Work out the finished part from the listing and answer in its coordinate system (mm). Face numbers are marked on the shaded views. A direction names the side the tool comes from. Coordinates: 2 decimals unless noted, no trailing zeros. Write each loop counter-clockwise with the first axis right and the second up, starting at its lowest first coordinate (ties: lowest second). Pieces come first, ordered by that corner, then holes. Notation, with made-up numbers: (2.5, -9.75) - (22.5, -9.75) arc R26 cw to (22.5, 8.25) - close; hole circle Ø8 at (-23, 84.25). An arc over 180 degrees is marked (long way). Use one line per item in the form item = value. Start each with the question number.
Item 1: A cutting plane is placed at B-B (z = 5). Write down the section's boundary in (x, y).
Item 2: For the marked faces 1 and 2, determine the directions among +Z, -Z, +X, -X, +Y, -Y from which every point of the face is accessible in a straight line to the end or side of a thin tool.
Item 3: Consider probe 1 along X at (y, z) = (-1.5, 5); probe 2 along Y at (x, z) = (-7.5, 7); probe 3 along Y at (x, z) = (1.5, 7.75). Determine where each line is inside the solid, lowest interval first.
Item 4: Given pin 1 (1 mm diameter, centred on x = 9.5, z = 6.5, fed in from -Y); pin 2 (1.8 mm diameter, centred on x = 2.5, z = 5, fed in from +Y) (3 decimals), each flat-ended and moving along its own axis, determine where each tip first touches the part or whether it passes through.
Item 5: A cutting plane is placed at A-A (y = 0). Write down the section's boundary in (x, z), then the cut area to 3 significant figures.
Item 6: A cutting plane is placed at C-C (x = -7.5). Write down the section's boundary in (y, z).
Item 7: A cutting plane is placed at D-D (y = -3.25). Write down the section's boundary in (x, z), then the cut area to 3 significant figures.
from build123d import *

# Parameters (mm, degrees)
SKETCH1_W           = 30
SKETCH1_H           = 10
BOSS_EXTRUDE1_DEPTH = 10
SKETCH2_R           = 1
CUT_EXTRUDE1_DEPTH  = 19.708286934
SKETCH4_R           = 1
CUT_EXTRUDE3_DEPTH  = 21.615528128
SKETCH3_R           = 1
BOSS_EXTRUDE2_DEPTH = 5


with BuildPart() as part:
    # Sketch1 → Boss-Extrude1 (new body)
    with BuildSketch(Plane.XY):
        Rectangle(SKETCH1_W, SKETCH1_H)
    extrude(amount=BOSS_EXTRUDE1_DEPTH)

    # Sketch2 → Cut-Extrude1 (cut, through all)
    with BuildSketch(Plane.XY.offset(10)):
        with Locations((-7.5, 0)):
            Circle(SKETCH2_R)
        with Locations((7.5, 0)):
            Circle(SKETCH2_R)
    extrude(amount=-CUT_EXTRUDE1_DEPTH, mode=Mode.SUBTRACT)

    # Sketch4 → Cut-Extrude3 (cut, through all)
    with BuildSketch(Plane(origin=(0, 5, 0), x_dir=(1, 0, 0), z_dir=(0, 1, 0))):
        with Locations(Location((-2.5, -5, 0), (0, 0, 270))):
            Circle(SKETCH4_R)
        with Locations(Location((2.5, -5, 0), (0, 0, 270))):
            Circle(SKETCH4_R)
    extrude(amount=-CUT_EXTRUDE3_DEPTH, mode=Mode.SUBTRACT)

    # Sketch3 → Boss-Extrude2 (add)
    with BuildSketch(Plane.XZ.offset(5)):
        with Locations(Location((13, 5, 0), (0, 0, 90))):
            Circle(SKETCH3_R)
    extrude(amount=BOSS_EXTRUDE2_DEPTH)


solid = part.part
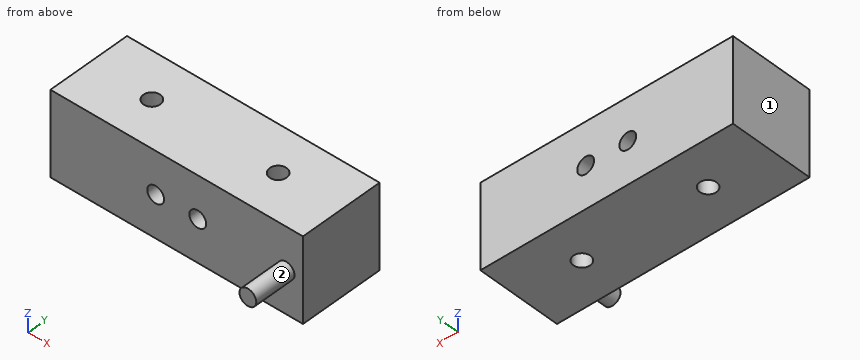
Answer:
q1.outline = (-15, -5) - (-3.5, -5) - (-3.5, 5) - (-15, 5) - close; (-1.5, -5) - (1.5, -5) - (1.5, 5) - (-1.5, 5) - close; (3.5, -5) - (12, -5) - (12, -10) - (14, -10) - (14, -5) - (15, -5) - (15, 5) - (3.5, 5) - close; hole circle Ø2 at (-7.5, 0); hole circle Ø2 at (7.5, 0)
q2.face_1 = +Z, -Z, -X, +Y, -Y
q2.face_2 = -Y
q3.probe_1 = -15 to -3.5, -1.5 to 1.5, 3.5 to 15
q3.probe_2 = -5 to -1, 1 to 5
q3.probe_3 = -5 to 5
q4.pin_1 = -5
q4.pin_2 = through
q5.outline = (-15, 0) - (-8.5, 0) - (-8.5, 10) - (-15, 10) - close; (-6.5, 0) - (6.5, 0) - (6.5, 10) - (-6.5, 10) - close; (8.5, 0) - (15, 0) - (15, 10) - (8.5, 10) - close; hole circle Ø2 at (-2.5, 5); hole circle Ø2 at (2.5, 5)
q5.area = 254 mm²
q6.outline = (-5, 0) - (-1, 0) - (-1, 10) - (-5, 10) - close; (1, 0) - (5, 0) - (5, 10) - (1, 10) - close
q7.outline = (-15, 0) - (15, 0) - (15, 10) - (-15, 10) - close; hole circle Ø2 at (-2.5, 5); hole circle Ø2 at (2.5, 5)
q7.area = 294 mm²
